from build123d import *

# Parameters (mm, degrees)
SKETCH5_W           = 12.880016042
SKETCH5_H           = 15.834691301
CUT_EXTRUDE2_DEPTH  = 7.62
CUT_EXTRUDE6_REACH  = 62
SKETCH11_W          = 3.175
SKETCH11_H          = 3.175
BOSS_EXTRUDE1_DEPTH = 6.35
CUT_EXTRUDE4_DEPTH  = 3.175
SKETCH10_W          = 4
SKETCH10_H          = 0.5
CUT_EXTRUDE5_DEPTH  = 37.349999944
CUT_EXTRUDE7_DEPTH  = 40.64
BOSS_EXTRUDE3_DEPTH = 12.7
SKETCH19_W          = 21.319602533
SKETCH19_H          = 36.10119369
CUT_EXTRUDE10_DEPTH = 13.7
SKETCH21_W          = 9.2375
SKETCH21_H          = 12.42619369
SKETCH21_H_2        = 3.175
BOSS_EXTRUDE4_DEPTH = 3.175
SKETCH17_W          = 3.175
SKETCH17_H          = 52.572237063
CUT_EXTRUDE9_DEPTH  = 20
CUT_EXTRUDE11_DEPTH = 4.175
CUT_EXTRUDE12_DEPTH = 2.625
FILLET1_R           = 2.54


with BuildPart() as part:
    # Sketch2 → Revolve1 (revolve)
    with BuildSketch(Plane(origin=(0, 0, 0), x_dir=(0, 0, -1), z_dir=(1, 0, 0))):
        Polygon((0, -50.8), (-29.999999944, 0), (0, 0), align=None)
    revolve(axis=Axis((0, 0, 0), (0, -1, 0)))

    # Sketch4 → Cut-Revolve1 (revolve, cut)
    with BuildSketch(Plane(origin=(0, 0, 0), x_dir=(0, 0, -1), z_dir=(1, 0, 0))):
        Polygon((0, -45.72), (-24.919999944, 0), (0, 0), align=None)
    revolve(axis=Axis((0, 16.11457811, 0), (0, -1, 0)), mode=Mode.SUBTRACT)

    # Sketch5 → Cut-Extrude2 (cut, symmetric)
    with BuildSketch(Plane(origin=(0, 0, 0), x_dir=(0, 0, -1), z_dir=(1, 0, 0))):
        with Locations((0, -47.812265381)):
            Rectangle(SKETCH5_W, SKETCH5_H)
    extrude(amount=CUT_EXTRUDE2_DEPTH, both=True, mode=Mode.SUBTRACT)

    # Sketch11 → Cut-Extrude6 (cut, up to next)
    with BuildSketch(Plane.XY.offset(29.999999944), mode=Mode.PRIVATE) as cut_extrude6_sk1:
        with Locations((4.7625, -1.5875)):
            Rectangle(SKETCH11_W, SKETCH11_H)
    cut_extrude6_tool1 = extrude(cut_extrude6_sk1.sketch, amount=-CUT_EXTRUDE6_REACH, mode=Mode.PRIVATE) & part.part
    add(cut_extrude6_tool1.solids().sort_by_distance((4.7625, -1.5875, 30))[0], mode=Mode.SUBTRACT)
    # Sketch11 → Cut-Extrude6 (cut, up to next)
    with BuildSketch(Plane.XY.offset(29.999999944), mode=Mode.PRIVATE) as cut_extrude6_sk2:
        with Locations((-4.7625, -1.5875)):
            Rectangle(SKETCH11_W, SKETCH11_H)
    cut_extrude6_tool2 = extrude(cut_extrude6_sk2.sketch, amount=-CUT_EXTRUDE6_REACH, mode=Mode.PRIVATE) & part.part
    add(cut_extrude6_tool2.solids().sort_by_distance((-4.7625, -1.5875, 30))[0], mode=Mode.SUBTRACT)

    # Sketch6 → Boss-Extrude1 (add, symmetric)
    with BuildSketch(Plane(origin=(0, 0, 0), x_dir=(0, 0, -1), z_dir=(1, 0, 0))):
        with BuildLine():
            Line((0, -39.89491973), (-7.374618631, -39.89491973))
            Line((-7.374618631, -39.89491973), (20.618728491, -87.296987611))
            ThreePointArc((20.618728491, -87.296987611), (38.876637468, -107.970587413), (63.5, -120.397935747))
            ThreePointArc((63.5, -120.397935747), (73.403024923, -122.48861576), (83.5, -123.19))
            Line((83.5, -123.19), (86.675, -123.19))
            Line((86.675, -123.19), (86.675, -115.2525))
            Line((86.675, -115.2525), (83.5, -115.2525))
            Line((83.5, -115.2525), (83.5, -116.84))
            ThreePointArc((83.5, -116.84), (50.445813134, -108.070287624), (26.086468861, -84.068007083))
            Line((26.086468861, -84.068007083), (0, -39.89491973))
        make_face()
        Polygon((-30.934610553, 0), (-7.374618631, -39.89491973), (0, -39.89491973), (-23.559991923, 0), align=None)
    extrude(amount=BOSS_EXTRUDE1_DEPTH, both=True)

    # Sketch7 → Cut-Extrude4 (cut)
    with BuildSketch(Plane(origin=(0, 0, 0), x_dir=(0, 0, -1), z_dir=(1, 0, 0))):
        with BuildLine():
            Line((-3.175, -39.89491973), (23.732438565, -85.458182452))
            ThreePointArc((23.732438565, -85.458182452), (45.650201216, -108.346121156), (75.457309, -119.106343424))
            ThreePointArc((75.457309, -119.106343424), (79.477830242, -119.567967375), (83.5, -120.015))
            Line((83.5, -120.015), (83.5, -116.84))
            ThreePointArc((83.5, -116.84), (50.445813134, -108.070287624), (26.086468861, -84.068007083))
            Line((26.086468861, -84.068007083), (-23.559991923, 0))
            Line((-23.559991923, 0), (-26.734991923, 0))
            Line((-26.734991923, 0), (-3.175, -39.89491973))
        make_face()
    cut_extrude4 = extrude(amount=-CUT_EXTRUDE4_DEPTH, mode=Mode.SUBTRACT)

    # Mirror1: Cut-Extrude4 across plane
    add(cut_extrude4.mirror(Plane(origin=(0, 0, 0), x_dir=(0, 0, 1), z_dir=(1, 0, 0))), mode=Mode.SUBTRACT)

    # Sketch9 → Cut-Revolve2 (revolve, cut)
    with BuildSketch(Plane(origin=(0, 0, 0), x_dir=(0, 0, -1), z_dir=(1, 0, 0))):
        Polygon((0, 0), (-24.9199908, 0), (-0.536470716, -39.89491973), (0, -39.89491973), align=None)
    revolve(axis=Axis((0, 16.11457811, 0), (0, -1, 0)), mode=Mode.SUBTRACT)

    # Sketch10 → Cut-Extrude5 (cut, through all)
    with BuildSketch(Plane.ZY.offset(6.35)):
        with BuildLine():
            Line((-79.5, -120.015), (-79.5, -116.719911574))
            ThreePointArc((-79.5, -116.719911574), (-81.499098876, -116.809971132), (-83.5, -116.84))
            Line((-83.5, -116.84), (-83.5, -120.015))
            Line((-83.5, -120.015), (-79.5, -120.015))
        make_face()
        with Locations((-81.5, -120.265)):
            Rectangle(SKETCH10_W, SKETCH10_H)
    extrude(amount=-CUT_EXTRUDE5_DEPTH, mode=Mode.SUBTRACT)

    # Sketch12 → Cut-Extrude7 (cut, symmetric)
    with BuildSketch(Plane.ZY):
        Polygon((30, 0), (-29.999999944, 0), (-29.999999944, -39.89491973), (-6.440008021, -39.89491973), (6.44000802, -39.89491973), align=None)
    extrude(amount=CUT_EXTRUDE7_DEPTH, both=True, mode=Mode.SUBTRACT)

    # Sketch18 → Boss-Extrude3 (add)
    with BuildSketch(Plane.ZY.offset(6.35)):
        with BuildLine():
            Line((6.44000802, -39.89491973), (6.44000802, -20.5))
            Line((6.44000802, -20.5), (9.61500802, -20.5))
            Line((9.61500802, -20.5), (9.61500802, -34.5185864))
            Line((9.61500802, -34.5185864), (9.61500802, -36.10119369))
            ThreePointArc((9.61500802, -36.10119369), (8.57844205, -39.89491973), (5.756782033, -42.634456374))
            Line((5.756782033, -42.634456374), (6.44000802, -41.477527034))
            Line((6.44000802, -41.477527034), (6.44000802, -39.89491973))
        make_face()
    extrude(amount=-BOSS_EXTRUDE3_DEPTH)

    # Sketch19 → Cut-Extrude10 (cut, through all)
    with BuildSketch(Plane.ZY.offset(6.35)):
        with Locations((20.274809287, -18.050596845)):
            Rectangle(SKETCH19_W, SKETCH19_H)
    extrude(amount=-CUT_EXTRUDE10_DEPTH, mode=Mode.SUBTRACT)

    # Sketch21 → Boss-Extrude4 (add)
    with BuildSketch(Plane.XY.offset(9.61500802)):
        with Locations((-10.96875, -29.888096845)):
            Rectangle(SKETCH21_W, SKETCH21_H)
        with Locations((10.96875, -29.888096845)):
            Rectangle(SKETCH21_W, SKETCH21_H)
        with Locations((10.96875, -22.0875)):
            Rectangle(SKETCH21_W, SKETCH21_H_2)
        with Locations((-10.96875, -22.0875)):
            Rectangle(SKETCH21_W, SKETCH21_H_2)
    extrude(amount=-BOSS_EXTRUDE4_DEPTH)

    # Sketch17 → Cut-Extrude9 (cut)
    with BuildSketch(Plane(origin=(0, 0, -86.675), x_dir=(-1, 0, 0), z_dir=(0, 0, -1))):
        with Locations((-4.7625, -96.903881469)):
            Rectangle(SKETCH17_W, SKETCH17_H)
        with Locations((4.7625, -96.903881469)):
            Rectangle(SKETCH17_W, SKETCH17_H)
    extrude(amount=-CUT_EXTRUDE9_DEPTH, mode=Mode.SUBTRACT)

    # Sketch22 → Cut-Extrude11 (cut, through all)
    with BuildSketch(Plane(origin=(0, 0, 6.44000802), x_dir=(-1, 0, 0), z_dir=(0, 0, -1))):
        Polygon((-15.5875, -24.405166536), (-15.5875, -36.10119369), (-8.680397482, -36.10119369), align=None)
        Polygon((15.5875, -24.405166536), (8.680397482, -36.10119369), (15.5875, -36.10119369), align=None)
    extrude(amount=-CUT_EXTRUDE11_DEPTH, mode=Mode.SUBTRACT)

    # Sketch24 → Cut-Extrude12 (cut, symmetric)
    with BuildSketch(Plane(origin=(0, 0, 0), x_dir=(0, 0, -1), z_dir=(1, 0, 0))):
        with BuildLine():
            Line((3.985949874, -59.1321491), (20.618728491, -87.296987611))
            ThreePointArc((20.618728491, -87.296987611), (40.186529767, -108.958439573), (66.675, -121.22539896))
            Line((66.675, -121.22539896), (66.675, -119.683023005))
            ThreePointArc((66.675, -119.683023005), (40.93327594, -107.645198887), (21.910320704, -86.534236305))
            Line((21.910320704, -86.534236305), (5.277542087, -58.369397794))
            Line((5.277542087, -58.369397794), (3.985949874, -59.1321491))
        make_face()
    extrude(amount=CUT_EXTRUDE12_DEPTH, both=True, mode=Mode.SUBTRACT)

    # Fillet1
    fillet1_edges = [part.edges().sort_by_distance(p)[0] for p in [
        (6.35, -64.965721992, -7.430973229),
        (6.35, -108.958439573, -40.186529767),
        (-6.35, -64.965721992, -7.430973229),
        (-6.35, -108.958439573, -40.186529767),
    ]]
    fillet(fillet1_edges, radius=FILLET1_R)


solid = part.part
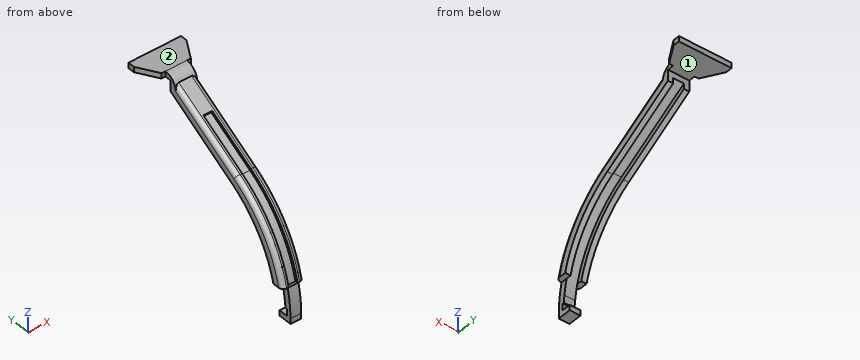
Geometry check sheet. Reference: the model listing, model coordinates, mm. Face numbers are marked on the shaded views. A direction names the side the tool comes from. Give positions to 0.01 mm unless a question says otherwise; leave off trailing zeros. Loops run counter-clockwise (first coordinate to the right, second up) from the corner with the lowest first, then second, coordinate; pieces in that order, holes last. Notation, with made-up numbers: (68, 47) -> (122, 47) arc R20 ccw to (122, 79) -> close; hole circle Ø8 at (51.25, 3). An arc over 180 degrees is marked (long way). Answer in a Markdown table with one row per item. Add a question column.
1) Cross-section at A-A on x = -5. Record the boundary of the cut face in (y, z) (3 decimals), and give its area (3 significant figures).
2) Cross-section at C-C on x = 11. Record the boundary of the cut face in (y, z) (3 decimals), and give its area (3 significant figures).
3) Cross-section at B-B on y = -38.5. Record the boundary of the cut face in (x, z), and give its area (3 significant figures).
4) Material ranges on probe 1 along X at (y, z) = (-99, -35.5) (3 decimals); probe 2 along X at (y, z) = (-101, -31.5) (3 decimals); probe 3 along Z at (x, y) = (2, -57), recorded low to high. Write a range as from..to.
5) Gauge pin test, flat ends, axial feed: P1, Ø3.5, axis at x = 5, y = -117.5, coming from the -Z side (3 decimals); P2, Ø4, axis at x = 1, y = -70.5, coming from the -Z side; P3, Ø0.5, axis at x = -0.5, y = -120.5, coming from the +Z side (3 decimals). Record the tip position at first contact, or that the pin passes through.
6) Set-up check for the marked faces 1 and 2: record each of +Z, -Z, +X, -X, +Y, -Y from which the full face is reachable in a straight line by a thin tool's end or side.
Outcome:
| question | item | result |
|---|---|---|
| 1 | outline | (-120.921, -66.675) -> (-114.682, -66.675) arc R66.678 cw to (-84.068, -26.086) -> (-39.895, 0) -> (-39.895, 6.44) -> (-20.5, 6.44) -> (-20.5, 9.615) -> (-36.101, 9.615) arc R7.461 ccw to (-42.881, 5.267) -> (-87.146, -20.874) arc R72.732 ccw to start |
| 1 | area | 720 mm^2 |
| 2 | outline | (-32.173, 6.44) -> (-20.5, 6.44) -> (-20.5, 9.615) -> (-32.173, 9.615) -> close |
| 2 | area | 37.1 mm^2 |
| 3 | outline | (-6.35, 6.44) -> (6.35, 6.44) -> (6.35, 9.22) -> (-6.35, 9.22) -> close |
| 3 | area | 35.3 mm^2 |
| 4 | probe 1 | x = -6.35..-3.175, 3.175..6.35 |
| 4 | probe 2 | x = -5.018..-2.625, 2.625..5.018 |
| 4 | probe 3 | z = -6.93..-2.73 |
| 5 | P1 | stops at z = -66.675 |
| 5 | P2 | stops at z = -16.08 |
| 5 | P3 | stops at z = -66.675 |
| 6 | face 1 | -Z, +X, -X, +Y |
| 6 | face 2 | +Z, +X, -X, +Y, -Y |
